from build123d import *

# Parameters (mm, degrees)
F1_DEPTH       = 1.5
F0_W           = 4
F0_H           = 33
F2_DEPTH       = 8
F3_W           = 33
F3_H           = 1.5
F4_DEPTH       = 0.5
F5_W           = 33
F5_H           = 1.5
F6_DEPTH       = 0.5
F7_W           = 2
F7_H           = 2
F8_DEPTH       = 2
F10_W          = 12
F10_H          = 24
F11_DEPTH      = 1.5
F13_DEPTH      = 25
F14_R          = 3
F9_R           = 2.35
F15_DEPTH      = 4
F16_DEPTH      = 2
F17_DEPTH      = 4
F17_DEPTH_BACK = 2
F18_DEPTH      = 0.2
F19_DEPTH      = 0.2
F20_DEPTH      = 0.2
F21_SIZE       = 0.5
F22_C1_SIZE    = 1.0999
F22_C2_SIZE    = 1.0999
F22_C3_SIZE    = 1.0999
F22_T7_DEPTH   = 9.637652322
F22_S8_R       = 2.35
F22_T9_DEPTH   = 6
F23_DEPTH      = 4.8
F24_SIZE       = 1.49999
F25_SIZE       = 2


# Not quite as in the source:
# - a fillet or chamfer that OpenCascade refuses, or shapes differently, is made with other operations: its cross-section is extruded or revolved along the edge and cut away or added
# - a fillet or chamfer is up to 0.001 mm smaller than in the source, because OpenCascade refuses the exact size


with BuildPart() as f1:
    # F0 (on Top) → F1 (new body)
    with BuildSketch(Plane.XY):
        Polygon((9.5, -16.5), (9.5, 16.5), (5, 16.5), (-5, 16.5), (-9.5, 16.5), (-9.5, -16.5), align=None)
    extrude(amount=F1_DEPTH)

    # F0 (on Top) → F2 (join)
    with BuildSketch(Plane.XY):
        with Locations((-11.5, 0)):
            Rectangle(F0_W, F0_H)
        with Locations((11.5, 0)):
            Rectangle(F0_W, F0_H)
    extrude(amount=F2_DEPTH)

    # F3 (on face) → F4 (cut)
    with BuildSketch(Plane.YZ.offset(-9.5)):
        with Locations((0, 4.25)):
            Rectangle(F3_W, F3_H)
    extrude(amount=-F4_DEPTH, mode=Mode.SUBTRACT)

    # F5 (on face) → F6 (cut)
    with BuildSketch(Plane(origin=(9.5, 0, 0), x_dir=(0, -1, 0), z_dir=(-1, 0, 0))):
        with Locations((0, 4.25)):
            Rectangle(F5_W, F5_H)
    extrude(amount=-F6_DEPTH, mode=Mode.SUBTRACT)

    # F7 (on face) → F8 (join)
    with BuildSketch(Plane.XY.offset(1.5)):
        with Locations((-8.5, 15.5)):
            Rectangle(F7_W, F7_H)
        with Locations((8.5, 15.5)):
            Rectangle(F7_W, F7_H)
        with Locations((8.5, -15.5)):
            Rectangle(F7_W, F7_H)
        with Locations((-8.5, -15.5)):
            Rectangle(F7_W, F7_H)
    extrude(amount=F8_DEPTH)

    # F10 (on face) → F11 (cut)
    with BuildSketch(Plane.XY.offset(1.5)):
        Rectangle(F10_W, F10_H)
    extrude(amount=-F11_DEPTH, mode=Mode.SUBTRACT)

    # F12 (on face) → F13 (cut)
    with BuildSketch(Plane.XY.offset(8)):
        Polygon((13.5, -6), (13.5, 6), (11.5, 6), (11.5, 0), (11.5, -6), align=None)
        Polygon((-11.5, 6), (-13.5, 6), (-13.5, -6), (-11.5, -6), (-11.5, 0), align=None)
    extrude(amount=-F13_DEPTH, mode=Mode.SUBTRACT)

    # F14
    f14_edges = [f1.edges().sort_by_distance(p)[0] for p in [
        (6, 12, 0.75),
        (-6, 12, 0.75),
        (-6, -12, 0.75),
        (6, -12, 0.75),
    ]]
    fillet(f14_edges, radius=F14_R)

    # F9 (on face) → F15 (join)
    with BuildSketch(Plane.XY.offset(8)):
        with BuildLine():
            Line((-9.5, 8.7600251258), (-9.5, 12.7399748742))
            ThreePointArc((-9.5, 12.7399748742), (-13.1, 10.75), (-9.5, 8.7600251258))
        make_face()
        with Locations((10.75, 10.75)):
            Circle(F9_R)
        with BuildLine():
            ThreePointArc((-8.4, -10.75), (-8.6933036199, -9.6131182999), (-9.5, -8.7600251258))
            Line((-9.5, -8.7600251258), (-9.5, -12.7399748742))
            ThreePointArc((-9.5, -12.7399748742), (-8.6933036199, -11.8868817001), (-8.4, -10.75))
        make_face()
        with Locations((10.75, -10.75)):
            Circle(F9_R)
    extrude(amount=F15_DEPTH)

    # F16 (add): faces of the model
    f16_faces = [f1.faces().sort_by_distance(p)[0] for p in [
        (9.0497739869, -10.75, 8),
        (9.0497739869, 10.75, 8),
    ]]
    extrude(f16_faces, amount=F16_DEPTH)

    # F9 (on face) → F17 (join, two sides)
    with BuildSketch(Plane.XY.offset(8)) as f17_sk:
        with BuildLine():
            ThreePointArc((-9.5, 8.7600251258), (-8.6933036199, 9.6131182999), (-8.4, 10.75))
            ThreePointArc((-8.4, 10.75), (-8.6933036199, 11.8868817001), (-9.5, 12.7399748742))
            Line((-9.5, 12.7399748742), (-9.5, 8.7600251258))
        make_face()
        with BuildLine():
            Line((-9.5, -12.7399748742), (-9.5, -8.7600251258))
            ThreePointArc((-9.5, -8.7600251258), (-13.1, -10.75), (-9.5, -12.7399748742))
        make_face()
        with BuildLine():
            ThreePointArc((-8.4, -10.75), (-8.6933036199, -9.6131182999), (-9.5, -8.7600251258))
            Line((-9.5, -8.7600251258), (-9.5, -12.7399748742))
            ThreePointArc((-9.5, -12.7399748742), (-8.6933036199, -11.8868817001), (-8.4, -10.75))
        make_face()
    extrude(amount=F17_DEPTH)
    extrude(f17_sk.sketch, amount=-F17_DEPTH_BACK)

    # F18 (add): faces of the model
    f18_faces = [f1.faces().sort_by_distance(p)[0] for p in [
        (-9.75, 0, 5),
        (9.75, 0, 5),
    ]]
    extrude(f18_faces, amount=F18_DEPTH)

    # F19 (add): a face of the model
    f19_faces = [f1.faces().sort_by_distance(p)[0] for p in [
        (-10, 0, 4.15),
    ]]
    extrude(f19_faces, amount=F19_DEPTH)

    # F20 (add): a face of the model
    f20_faces = [f1.faces().sort_by_distance(p)[0] for p in [
        (10, 0, 4.15),
    ]]
    extrude(f20_faces, amount=F20_DEPTH)

    # F21
    f21_edges = [f1.edges().sort_by_distance(p)[0] for p in [
        (8.4, 10.75, 12),
        (8.4, -10.75, 12),
        (-13.1, -10.75, 12),
        (-13.1, 10.75, 12),
        (-8.4, 10.75, 12),
        (-8.4, -10.75, 12),
    ]]
    chamfer(f21_edges, length=F21_SIZE)

    # F22: chamfer of 1.1 on 4 edges, made by hand

    # F22_c1 (size 1.1 in the source; OpenCascade refuses exactly that, so slightly less here)
    f22_c1_edges = [f1.edges().sort_by_distance(p)[0] for p in [
        (9.5, 10.75, 6),
    ]]
    chamfer(f22_c1_edges, length=F22_C1_SIZE)

    # F22_c2 (size 1.1 in the source; OpenCascade refuses exactly that, so slightly less here)
    f22_c2_edges = [f1.edges().sort_by_distance(p)[0] for p in [
        (9.5, -10.75, 6),
    ]]
    chamfer(f22_c2_edges, length=F22_C2_SIZE)

    # F22_c3 (size 1.1 in the source; OpenCascade refuses exactly that, so slightly less here)
    f22_c3_edges = [f1.edges().sort_by_distance(p)[0] for p in [
        (-9.5, 10.75, 6),
    ]]
    chamfer(f22_c3_edges, length=F22_C3_SIZE)


with BuildPart() as f22_tool5:
    # F22_s6 → F22_t7 (new body)
    with BuildSketch(Plane.XZ.offset(15.568826161)):
        with BuildLine():
            Line((-9.5311126984, 4.8688873016), (-8.3688873016, 6.0311126984))
            Line((-8.3688873016, 6.0311126984), (-8.3688873016, 6.0531126984))
            ThreePointArc((-8.3688873016, 6.0531126984), (-8.9344436508, 6.022), (-9.5, 6.022))
            Line((-9.5, 6.022), (-9.522, 6))
            ThreePointArc((-9.522, 6), (-9.522, 5.4344436508), (-9.5531126984, 4.8688873016))
            Line((-9.5531126984, 4.8688873016), (-9.5311126984, 4.8688873016))
        make_face()
    extrude(amount=-F22_T7_DEPTH)

    # F22_s8 → F22_t9 (intersect, symmetric)
    with BuildSketch(Plane.XY.offset(5.5)):
        with Locations((-10.75, -10.75)):
            Circle(F22_S8_R)
    extrude(amount=F22_T9_DEPTH, both=True, mode=Mode.INTERSECT)


with BuildPart() as f1_1:
    add(f1.part)

    # F22_t4: union F22_tool5
    add(f22_tool5.part)

    # F0 (on Top) → F23 (join, through all)
    with BuildSketch(Plane.XY):
        Polygon((-5, 16.5), (5, 16.5), (5, 18), (0, 18), (-5, 18), align=None)
    extrude(amount=F23_DEPTH)

    # F24 (size 1.5 in the source; OpenCascade refuses exactly that, so slightly less here)
    f24_edges = [f1_1.edges().sort_by_distance(p)[0] for p in [
        (-5, 18, 2.4),
        (5, 18, 2.4),
    ]]
    chamfer(f24_edges, length=F24_SIZE)

    # F25
    f25_edges = [f1_1.edges().sort_by_distance(p)[0] for p in [
        (13.5, -16.5, 4),
        (-13.5, -16.5, 4),
        (13.5, 16.5, 4),
        (-13.5, 16.5, 4),
    ]]
    chamfer(f25_edges, length=F25_SIZE)


solid = f1_1.part
Part model, mm, in its own coordinate system. A direction names the side the tool comes from. Give positions to 0.01 mm unless a question says otherwise; leave off trailing zeros. Loops run counter-clockwise (first coordinate to the right, second up) from the corner with the lowest first, then second, coordinate; pieces in that order, holes last.
(1) Band-saw the part on A-A (z = 2.5). Count the separate pieces of the cut face and the enclosed holes in it, and give its area (3 significant figures).
Return value:
separate pieces: 3
enclosed holes: 0
area: 237 mm2
(2) Band-saw the part on D-D (x = 10.75). Write the cut outline in (y, z), and give its area (3 significant figures).
Return value:
outline: (-16.5, 0) - (16.5, 0) - (16.5, 8) - (13.1, 8) - (13.1, 11.5) - (12.6, 12) - (8.9, 12) - (8.4, 11.5) - (8.4, 8) - (-8.4, 8) - (-8.4, 11.5) - (-8.9, 12) - (-12.6, 12) - (-13.1, 11.5) - (-13.1, 8) - (-16.5, 8) - close
area: 301 mm2
(3) 3-axis set-ups, long thin cutter, end or side, ignore diameter. For faces 1 (the flat face through (-9, 14.5, 2)), 2 (the flat face through (-7.5, 15, 2)), 3 (the flat face through (13, 6, 4)), 4 (the flat face through (-13.5, 10, 4)), 5 (the flat face through (0, -12, 1)): which of +Z, -Z, +X, -X, +Y, -Y reach the whole face in a straight line?
Return value:
face 1: +Z
face 2: +Z, +Y, -Y
face 3: +Z, -Z, +X
face 4: +Z, -Z, -X, +Y, -Y
face 5: +Z, -Z
(4) Drill centre lines: line 1 along X through (y, z) = (-7, 5.25); line 2 along X through (y, z) = (-12, 9.75); line 3 along Y through (x, z) = (-7.75, 2.5). Where is each one in solid material? Low to high.
Return value:
line 1: x = -13.5 to -9.5, 9.5 to 13.5
line 2: x = -12.74 to -8.76, 8.76 to 12.74
line 3: y = -16.5 to -14.5, 14.5 to 16.5
(5) Band-saw the part on C-C (z = 6.5). Write the cut outline in (x, y).
Return value:
outline: (-13.5, -14.5) - (-11.5, -16.5) - (-9.5, -16.5) - (-9.5, -12.74) arc R2.35 ccw to (-9.5, -8.76) - (-9.5, 8.76) arc R2.35 ccw to (-9.5, 12.74) - (-9.5, 16.5) - (-11.5, 16.5) - (-13.5, 14.5) - (-13.5, 6) - (-11.5, 6) - (-11.5, -6) - (-13.5, -6) - close; (9.5, -16.5) - (11.5, -16.5) - (13.5, -14.5) - (13.5, -6) - (11.5, -6) - (11.5, 6) - (13.5, 6) - (13.5, 14.5) - (11.5, 16.5) - (9.5, 16.5) - (9.5, 12.74) arc R2.35 ccw to (9.5, 8.76) - (9.5, -8.76) arc R2.35 ccw to (9.5, -12.74) - close
(6) Band-saw the part on B-B (x = -0.75). Write the cut outline in (y, z), and give its area (3 significant figures).
Return value:
outline: (-16.5, 0) - (-12, 0) - (-12, 1.5) - (-16.5, 1.5) - close; (12, 0) - (18, 0) - (18, 4.8) - (16.5, 4.8) - (16.5, 1.5) - (12, 1.5) - close
area: 20.7 mm2
(7) Pin check, flat tips, straight feed: pin 1 (0.6 mm diameter, centred on y = -15, z = 2, fed in from -X); pin 2 (0.6 mm diameter, centred on x = -12.5, z = 3, fed in from +Y); pin 3 (2 mm diameter, centred on x = -6.5, y = -7, fed in from -Z); pin 4 (1 mm diameter, centred on x = -12.5, z = 3.5, fed in from -Y). Stop position of each tip, or through.
Return value:
pin 1: stops at x = -13.3
pin 2: stops at y = 15.8
pin 3: stops at z = 0
pin 4: stops at y = -16
(8) Pull direction Z, two halves, no side cores. Call faces 6 (the flat face through (11, 0, 8)), 7 (the flat face through (-6.2, 1, 0)), 8 (the flat face through (9, 16.5, 3)), 9 (the flat face through (9.1, -10.8, 5.3)): pulls with the +Z half, pulls with the -Z half, needs draft (parallel to the pull), parting line crosses it, or undercut.
Return value:
face 6: pulls with the +Z half
face 7: pulls with the -Z half
face 8: needs draft
face 9: undercut
